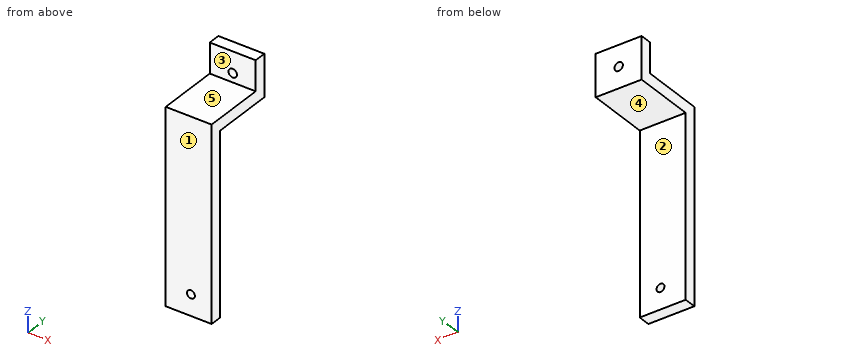
```python
from build123d import *

# Parameters (mm, degrees)
EXTRUDE_THIN1_DEPTH = 38.1
SKETCH2_R           = 3.5
CUT_EXTRUDE1_DEPTH  = 199.45691472
SKETCH4_R           = 3.3
CUT_EXTRUDE3_DEPTH  = 60


with BuildPart() as part:
    # Sketch1 → Extrude-Thin1 (new body)
    with BuildSketch(Plane(origin=(0, 0, 0), x_dir=(0, 0, -1), z_dir=(1, 0, 0))):
        Polygon((0, 0), (34.93, 0), (34.93, -51.11), (184.93, -51.11), (184.93, -61.11), (24.93, -61.11), (24.93, -10), (0, -10), align=None)
    extrude(amount=EXTRUDE_THIN1_DEPTH)

    # Sketch2 → Cut-Extrude1 (cut, through all)
    with BuildSketch(Plane(origin=(0, 0, 0), x_dir=(1, 0, 0), z_dir=(0, 1, 0))):
        with Locations(Location((19.05, 17.465, 0), (0, 0, 270))):
            Circle(SKETCH2_R)
    extrude(amount=-CUT_EXTRUDE1_DEPTH, mode=Mode.SUBTRACT)

    # Sketch4 → Cut-Extrude3 (cut)
    with BuildSketch(Plane(origin=(0, -51.11, 0), x_dir=(1, 0, 0), z_dir=(0, 1, 0))):
        with Locations(Location((20.897590421, 167.59354, 0), (0, 0, 270))):
            Circle(SKETCH4_R)
    extrude(amount=-CUT_EXTRUDE3_DEPTH, mode=Mode.SUBTRACT)


solid = part.part
```
The listing builds one solid part. Answer for the finished solid, in the listing's coordinates (mm). Face numbers are marked on the shaded views. A direction names the side the tool comes from. Round coordinates to 2 decimals unless told otherwise and drop trailing zeros. Order: outer loops, then holes, each group sorted by start corner. A loop starts at its lowest first (then second) coordinate and runs counter-clockwise, first axis right, second up. Notation, with made-up numbers: (56.5, 59.5) - (77.5, 59.5) arc R21 ccw to (77.5, 66.5) - close; hole circle Ø7 at (-7, 56). An arc over 180 degrees is marked (long way). Put each result on its own line as item: value. Start each with the question number.
(1) Find section B-B (z = -141.5). Give the vertices of the cut face in (x, y), plus the area to 3 significant figures.
(2) Straight lines are drawn through the part: probe 1 along Z at (x, y) = (17, -33); probe 2 along Y at (x, z) = (16.5, -113); probe 3 along Y at (x, z) = (11, -17.5). For each, find the intervals that lie inside material, in ascending order. Write a range as from..to.
(3) Find section C-C (y = -34.5). Give the vertices of the cut face in (x, z), plus the area to 3 significant figures.
(4) Given P1, Ø4, axis at x = 20, y = -25, coming from the -Z side; P2, Ø11.5, axis at x = 13.5, y = -43, coming from the +Z side; P3, Ø1, axis at x = 23, z = -20, coming from the -Y side, each flat-ended and moving along its own axis, determine where each tip first touches the part or whether it passes through.
(5) For the marked faces 1 and 2, determine the directions among +Z, -Z, +X, -X, +Y, -Y from which every point of the face is accessible in a straight line to the end or side of a thin tool.
(6) Determine the mould class of the marked faces 3, 4 and 5 for opening direction Z: released by +Z, released by -Z, zero draft, split by the parting line, or undercut.
(7) Find section A-A (x = 6). Give the vertices of the cut face in (y, z), plus the area to 3 significant figures.
Reply:
1. outline: (0, -61.11) - (38.1, -61.11) - (38.1, -51.11) - (0, -51.11) - close
1. area: 381 mm^2
2. probe 1: -34.93..-24.93
2. probe 2: -61.11..-51.11
2. probe 3: -10..0
3. outline: (0, -34.93) - (38.1, -34.93) - (38.1, -24.93) - (0, -24.93) - close
3. area: 381 mm^2
4. P1: z = -34.93
4. P2: z = -24.93
4. P3: y = -10
5. face 1: +Z, -Z, +X, -X, -Y
5. face 2: -Z, +X, -X, +Y
6. face 3: zero draft
6. face 4: released by -Z
6. face 5: released by +Z
7. outline: (-61.11, -184.93) - (-51.11, -184.93) - (-51.11, -34.93) - (0, -34.93) - (0, 0) - (-10, 0) - (-10, -24.93) - (-61.11, -24.93) - close
7. area: 2,360 mm^2
